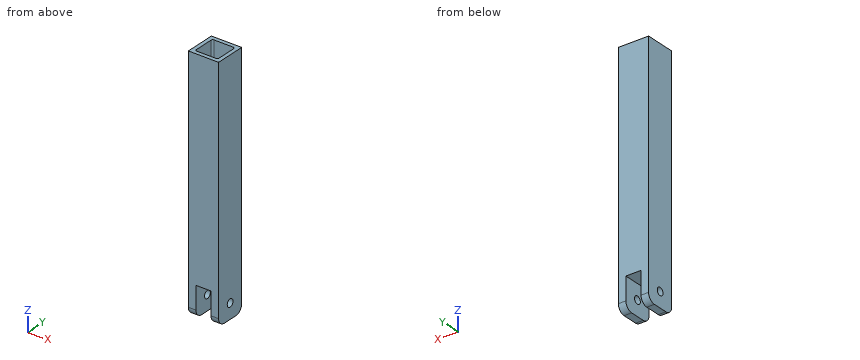
```python
from build123d import *

# Parameters (mm, degrees)
F0_W     = 200
F0_H     = 1600
F1_DEPTH = 200
F2_W     = 100
F2_H     = 200
F3_DEPTH = 400
F4_W     = 150
F4_H     = 150
F5_DEPTH = 500
F6_R     = 25
F7_DEPTH = 300
F8_R     = 10
F9_R     = 50


with BuildPart() as f1:
    # F0 (on Right) → F1 (new body)
    with BuildSketch(Plane.YZ):
        with Locations((100, 800)):
            Rectangle(F0_W, F0_H)
    extrude(amount=F1_DEPTH)

    # F2 (on face) → F3 (cut)
    with BuildSketch(Plane(origin=(0, 200, 0), x_dir=(-1, 0, 0), z_dir=(0, 1, 0))):
        with Locations((-100, 100)):
            Rectangle(F2_W, F2_H)
    extrude(amount=-F3_DEPTH, mode=Mode.SUBTRACT)

    # F4 (on face) → F5 (cut)
    with BuildSketch(Plane.XY.offset(1600)):
        with Locations((100, 100)):
            Rectangle(F4_W, F4_H)
    extrude(amount=-F5_DEPTH, mode=Mode.SUBTRACT)

    # F6 (on face) → F7 (cut)
    with BuildSketch(Plane(origin=(0, 0, 0), x_dir=(0, -1, 0), z_dir=(-1, 0, 0))):
        with Locations((-100, 100)):
            Circle(F6_R)
    extrude(amount=-F7_DEPTH, mode=Mode.SUBTRACT)

    # F8
    f8_edges = [f1.edges().sort_by_distance(p)[0] for p in [
        (25, 175, 1350),
        (175, 175, 1350),
        (25, 25, 1350),
        (175, 25, 1350),
    ]]
    fillet(f8_edges, radius=F8_R)

    # F9
    f9_edges = [f1.edges().sort_by_distance(p)[0] for p in [
        (175, 200, 0),
        (25, 200, 0),
        (25, 0, 0),
        (175, 0, 0),
    ]]
    fillet(f9_edges, radius=F9_R)


solid = f1.part
```
Geometry: final body of the model. Coordinates: model frame, mm. Round coordinates to 2 decimals unless told otherwise and drop trailing zeros. Order: outer loops, then holes, each group sorted by start corner. A loop starts at its lowest first (then second) coordinate and runs counter-clockwise, first axis right, second up. Notation, with made-up numbers: (-5, 17.25) -> (22, 17.25) arc R19 cw to (22, 54.25) -> close; hole circle Ø1 at (58.25, 89.25). An arc over 180 degrees is marked (long way). Use CSV: the item, a comma, the result in double quotes. Start each with the question number.
1) Section D-D (x = 122.5). Return the cut outline in (y, z), and give its area (3 significant figures).
2) Section B-B (z = 1439). Return the cut outline in (x, y).
3) First-contact query: pin 1 Ø1.5 at (x, y) = (51, 61.5) entering from -Z; pin 2 Ø5 at (x, y) = (150.5, 140.5) entering from +Z. Flat tips, straight axial feed; report the tip coordinate or a pass-through.
4) Section A-A (y = 100). Return the cut outline in (x, z), and give its area (3 significant figures).
5) Section C-C (z = 100). Return the cut outline in (x, y).
6) Material intervals for line 1 along Z through (x, y) = (16, 100); line 2 along Y through (x, z) = (159, 1140.5), sorted ascending. Write a range as from..to.
Returned:
1,outline,"(0, 200) -> (200, 200) -> (200, 1600) -> (175, 1600) -> (175, 1100) -> (25, 1100) -> (25, 1600) -> (0, 1600) -> close"
1,area,"205,000 mm²"
2,outline,"(0, 0) -> (200, 0) -> (200, 200) -> (0, 200) -> close; hole (25, 35) arc R10 ccw to (35, 25) -> (165, 25) arc R10 ccw to (175, 35) -> (175, 165) arc R10 ccw to (165, 175) -> (35, 175) arc R10 ccw to (25, 165) -> close"
3,pin 1,"stops at z = 200"
3,pin 2,"stops at z = 1100"
4,outline,"(0, 0) -> (50, 0) -> (50, 75) -> (0, 75) -> close; (0, 125) -> (50, 125) -> (50, 200) -> (150, 200) -> (150, 125) -> (200, 125) -> (200, 1600) -> (175, 1600) -> (175, 1100) -> (25, 1100) -> (25, 1600) -> (0, 1600) -> close; (150, 0) -> (200, 0) -> (200, 75) -> (150, 75) -> close"
4,area,"220,000 mm²"
5,outline,"(0, 0) -> (50, 0) -> (50, 75) -> (0, 75) -> close; (0, 125) -> (50, 125) -> (50, 200) -> (0, 200) -> close; (150, 0) -> (200, 0) -> (200, 75) -> (150, 75) -> close; (150, 125) -> (200, 125) -> (200, 200) -> (150, 200) -> close"
6,line 1,"z = 0..75, 125..1600"
6,line 2,"y = 0..25, 175..200"
